For this review, take the finished solid that the model builds, in its own axes (mm). Face numbers are marked on the shaded views. A direction names the side the tool comes from. Round coordinates to 2 decimals unless told otherwise and drop trailing zeros. Order: outer loops, then holes, each group sorted by start corner. A loop starts at its lowest first (then second) coordinate and runs counter-clockwise, first axis right, second up. Notation, with made-up numbers: (-0.5, -4) -> (24.5, -4) arc R31 cw to (24.5, 34) -> close; hole circle Ø8 at (50, -20.75). An arc over 180 degrees is marked (long way). Use a Markdown table: item, result. Add a question column.
1) Consider section C-C (z = 60). State the section outline as (x, y) points, plus the area to 3 significant figures.
2) Wall thickness on line 1 along X through (y, z) = (-124, 28.5); line 2 along Y through (x, z) = (-58, 30); line 3 along Z through (x, y) = (83.5, -96.5): over which ranges is each line inside the solid? List them lowest first. Write a range as [from, to].
3) Consider section D-D (z = 30). State the section outline as (x, y) points.
4) Consider section A-A (x = -93). State the section outline as (y, z) points.
5) Machinability: for the marked faces 4 and 5, which of the approach directions +Z, -Z, +X, -X, +Y, -Y give a long, thin tool a straight path to every point of the face, cutting with its end or side? Answer none if there is none.
6) Clearance check with a flat-ended pin moving along its axis: P1, Ø10, axis at x = -51, y = -173, coming from the -Z side. State where the tip first meets the part, or that it passes through.
7) Consider section B-B (y = -72). State the section outline as (x, z) points, plus the area to 3 significant figures.
8) Draft analysis for pull direction X (two halves, no side actions). For the marked faces 1, 2 and 3, state which applies: pulls with the +X half, pulls with the -X half, needs draft (parallel to the pull), parting line crosses it, or undercut.
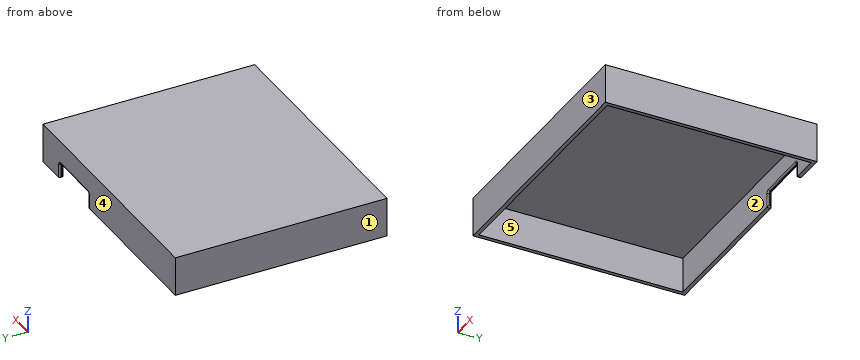
```python
from build123d import *

# Parameters (mm, degrees)
F0_W     = 320
F0_H     = 50
F1_DEPTH = 270
F2_T     = -5
F3_W     = 70
F3_H     = 20
F4_DEPTH = 25
F5_F1_R  = 2
F5_F2_R  = 2


with BuildPart() as f1:
    # F0 (on Front) → F1 (new body)
    with BuildSketch(Plane.XZ):
        with Locations((-36.4068159834, 46.1331414707)):
            Rectangle(F0_W, F0_H)
    extrude(amount=F1_DEPTH)

    # F2
    f2_openings = [f1.faces().sort_by_distance(p)[0] for p in [
        (-36.406816, -135, 21.133141),
    ]]
    offset(amount=F2_T, openings=f2_openings)

    # F3 (on face) → F4 (cut)
    with BuildSketch(Plane(origin=(0, 0, 0), x_dir=(-1, 0, 0), z_dir=(0, 1, 0))):
        with Locations((-48.5931840166, 31.1331414707)):
            Rectangle(F3_W, F3_H)
    extrude(amount=-F4_DEPTH, mode=Mode.SUBTRACT)

    # F5: fillet of radius 2 on 6 edges, made by hand

    # F5_f1
    f5_f1_edges = [f1.edges().sort_by_distance(p)[0] for p in [
        (83.5931840166, -2.5, 41.1331414707),
        (13.5931840166, -2.5, 41.1331414707),
    ]]
    fillet(f5_f1_edges, radius=F5_F1_R)

    # F5_f2
    f5_f2_edges = [f1.edges().sort_by_distance(p)[0] for p in [
        (83.5931840166, -2.5, 21.1331414707),
        (13.5931840166, -2.5, 21.1331414707),
        (48.5931840166, 0, 41.1331414707),
        (48.5931840166, -5, 41.1331414707),
        (83.007397579, -5, 40.5473550331),
        (14.1789704543, -5, 40.5473550331),
        (14.1789704543, 0, 40.5473550331),
        (83.007397579, 0, 40.5473550331),
    ]]
    fillet(f5_f2_edges, radius=F5_F2_R)


solid = f1.part
```
Results list:
| question | item | result |
|---|---|---|
| 1 | outline | (-196.41, -270) -> (123.59, -270) -> (123.59, 0) -> (-196.41, 0) -> close; hole (-191.41, -265) -> (118.59, -265) -> (118.59, -5) -> (-191.41, -5) -> close |
| 1 | area | 5,800 mm2 |
| 2 | line 1 | [-196.41, -191.41], [118.59, 123.59] |
| 2 | line 2 | [-270, -265], [-5, 0] |
| 2 | line 3 | [66.13, 71.13] |
| 3 | outline | (-196.41, -270) -> (123.59, -270) -> (123.59, 0) -> (85.59, 0) arc R2 ccw to (83.59, -2) -> (83.59, -3) arc R2 ccw to (85.59, -5) -> (118.59, -5) -> (118.59, -265) -> (-191.41, -265) -> (-191.41, -5) -> (11.59, -5) arc R2 ccw to (13.59, -3) -> (13.59, -2) arc R2 ccw to (11.59, 0) -> (-196.41, 0) -> close |
| 4 | outline | (-270, 21.13) -> (-265, 21.13) -> (-265, 66.13) -> (-5, 66.13) -> (-5, 21.13) -> (0, 21.13) -> (0, 71.13) -> (-270, 71.13) -> close |
| 5 | face 4 | +Z, -Z, +X, -X, +Y |
| 5 | face 5 | -Z |
| 6 | P1 | z = 66.13 |
| 7 | outline | (-196.41, 21.13) -> (-191.41, 21.13) -> (-191.41, 66.13) -> (118.59, 66.13) -> (118.59, 21.13) -> (123.59, 21.13) -> (123.59, 71.13) -> (-196.41, 71.13) -> close |
| 7 | area | 2,050 mm2 |
| 8 | face 1 | pulls with the -X half |
| 8 | face 2 | undercut |
| 8 | face 3 | needs draft |
